The listing builds one solid part. Answer for the finished solid, in the listing's coordinates (mm). A direction names the side the tool comes from. Give positions to 0.01 mm unless a question says otherwise; leave off trailing zeros. Order: outer loops, then holes, each group sorted by start corner. A loop starts at its lowest first (then second) coordinate and runs counter-clockwise, first axis right, second up. Notation, with made-up numbers: (-21.75, 59) - (25.25, 59) arc R22 ccw to (25.25, 71) - close; hole circle Ø1 at (21.25, 11). An arc over 180 degrees is marked (long way). Use a Markdown table: item, result. Add a question column.
1) Find section D-D, the plane x = 103. Determine the outline of the cut face in (y, z).
2) Flat-ended cylindrical pins translate along their axes: pin 1 (3 mm diameter, centred on x = 62, z = 39.5, fed in from -Y); pin 2 (6 mm diameter, centred on x = 18, y = 60, fed in from +Z); pin 3 (5 mm diameter, centred on y = 25, z = 45.5, fed in from +X). Find the tip coordinate at first contact, or state that the pin passes through.
3) For faces 1 (the face through (47.64, 69.74, 63.19)), 2 (the face through (10.56, 99.85, 54.58)), 3 (the face through (95.313, 14.897, 33.217)), 4 (the face through (39.38, 63.86, 63.19)), determine the directions among +Z, -Z, +X, -X, +Y, -Y from which every point of the face is accessible in a straight line to the end or side of a thin tool.
4) Straight lines are drawn through the part: line 1 (Z direction, x = 30.5, y = 19.5); line 2 (Y direction, x = 71, z = 53); line 3 (X direction, y = 98.5, z = 67.5). For each, find the intervals that lie inside material, in ascending order.
5) Find section C-C, the plane y = 36. Determine the outline of the cut face in (x, z).
6) Find section A-A, the plane z = 93.5. Determine the outline of the cut face in (x, y).
7) The mould has two halves that part along Z. Classify faces 5 (the face through (40.316, 70.091, 100.864)), 6 (the face through (110, 54, 12)), 7 (the face through (42, 56, 25)): released by +Z, released by -Z, zero draft, split by the parting line, or undercut.
8) Find section B-B, the plane z = 29. Determine the outline of the cut face in (x, y).
from build123d import *

# Parameters (mm, degrees)
F0_W     = 110
F0_H     = 110
F1_DEPTH = 25
F3_DEPTH = 120
F4_R     = 16
F5_DEPTH = 25


with BuildPart() as f1:
    # F0 (on Top) → F1 (new body)
    with BuildSketch(Plane.XY):
        with Locations((55, 55)):
            Rectangle(F0_W, F0_H)
    extrude(amount=F1_DEPTH)

    # F2 (on face) → F3 (join)
    with BuildSketch(Plane.XY.offset(25)):
        Polygon((14.045202, 103.334524), (6.974134, 96.263456), (91.826948, 11.410642), (98.898016, 18.48171), align=None)
    extrude(amount=F3_DEPTH)

    # F4 (on face) → F5 (cut)
    with BuildSketch(Plane(origin=(58.689863, 58.689863, 0), x_dir=(-0.707107, 0.707107, 0), z_dir=(0.707107, 0.707107, 0))):
        with BuildLine():
            ThreePointArc((-8.862915, 109), (35.786196, 122.947332), (63.137085, 85))
            Line((63.137085, 85), (63.246235, 158.167794))
            Line((63.246235, 158.167794), (-56.862915, 158.167794))
            Line((-56.862915, 158.167794), (-56.862915, 41.666667))
            ThreePointArc((-56.862915, 41.666667), (-56.349748, 44.828944), (-54.862915, 47.666667))
            Line((-54.862915, 47.666667), (-8.862915, 109))
        make_face()
        with Locations((23.137085, 85)):
            Circle(F4_R)
    extrude(amount=-F5_DEPTH, mode=Mode.SUBTRACT)


solid = f1.part
The answers:
| question | item | result |
|---|---|---|
| 1 | outline | (0, 0) - (110, 0) - (110, 25) - (0, 25) - close |
| 2 | pin 1 | y = 39.74 |
| 2 | pin 2 | z = 25 |
| 2 | pin 3 | x = 94.88 |
| 3 | face 1 | +Z, +X, +Y |
| 3 | face 2 | +Z, -X, +Y |
| 3 | face 3 | +Z, +X, -Y |
| 3 | face 4 | +Z, -X, -Y |
| 4 | line 1 | 0 to 25 |
| 4 | line 2 | 32.24 to 46.38 |
| 4 | line 3 | 9.21 to 18.88 |
| 5 | outline | (0, 0) - (110, 0) - (110, 25) - (81.38, 25) - (81.38, 78.03) - (67.24, 91.37) - (67.24, 25) - (0, 25) - close |
| 6 | outline | (7.62, 95.62) - (25.67, 77.56) - (32.74, 84.64) - (14.69, 102.69) - close; (44.84, 58.39) - (66.11, 37.13) - (73.18, 44.2) - (51.91, 65.47) - close |
| 7 | face 5 | undercut |
| 7 | face 6 | zero draft |
| 7 | face 7 | released by +Z |
| 8 | outline | (6.97, 96.26) - (91.83, 11.41) - (98.9, 18.48) - (14.05, 103.33) - close |
